from build123d import *

# Parameters (mm, degrees)
SKETCH1_W                   = 1212.85
SKETCH1_H                   = 736.6
BOSS_EXTRUDE1_DEPTH         = 6.35
H_0_266_DIAMETER_HOLE1_D    = 6.7564
H_0_266_DIAMETER_HOLE2_D    = 6.7564
H_0_266_DIAMETER_HOLE3_D    = 6.7564
SKETCH12_R                  = 3.175
CUT_EXTRUDE4_DEPTH          = 7.35
LPATTERN1_COUNT             = 5
LPATTERN1_PITCH             = 266.7
FILLET2_R                   = 3.175
CUT_EXTRUDE5_DEPTH          = 7.35
F_1_4_0_25_DIAMETER_HOLE1_D = 6.35


with BuildPart() as part:
    # Sketch1 → Boss-Extrude1 (new body)
    with BuildSketch(Plane.XY):
        Rectangle(SKETCH1_W, SKETCH1_H)
    extrude(amount=BOSS_EXTRUDE1_DEPTH)

    # H (0.266) Diameter Hole1 (through all)
    with Locations(Plane.XY.offset(6.35)):
        with Locations((-565.15, -342.9), (-158.75, -342.9), (247.65, -342.9)):
            Hole(H_0_266_DIAMETER_HOLE1_D / 2)

    # H (0.266) Diameter Hole2 (through all)
    with Locations(Plane.XY.offset(6.35)):
        with Locations((-582.6125, 323.596), (-582.6125, 171.196), (-582.6125, 18.796), (-582.6125, -133.604)):
            Hole(H_0_266_DIAMETER_HOLE2_D / 2)

    # H (0.266) Diameter Hole3 (through all)
    with Locations(Plane.XY.offset(6.35)):
        with Locations((223.770762516, 324.305909426), (436.157706379, 167.711380386), (301.059782944, 190.437399177)):
            Hole(H_0_266_DIAMETER_HOLE3_D / 2)

    # Sketch12 → Cut-Extrude4 (cut, through all)
    with BuildSketch(Plane.XY.offset(6.35)):
        with Locations((-536.575, 361.95)):
            Circle(SKETCH12_R)
        with BuildLine():
            Line((-552.45, 355.6), (-520.7, 355.6))
            ThreePointArc((-520.7, 355.6), (-508, 342.9), (-520.7, 330.2))
            Line((-520.7, 330.2), (-552.45, 330.2))
            ThreePointArc((-552.45, 330.2), (-565.15, 342.9), (-552.45, 355.6))
        make_face()
    cut_extrude4 = extrude(amount=-CUT_EXTRUDE4_DEPTH, mode=Mode.SUBTRACT)

    # LPattern1: Cut-Extrude4 ×5
    with Locations(*[(i * LPATTERN1_PITCH, 0, 0) for i in range(1, LPATTERN1_COUNT)]):
        add(cut_extrude4, mode=Mode.SUBTRACT)

    # Fillet2
    fillet2_edges = [part.edges().sort_by_distance(p)[0] for p in [
        (606.425, -368.3, 3.175),
        (-606.425, -368.3, 3.175),
        (-606.425, 368.3, 3.175),
        (606.425, 368.3, 3.175),
    ]]
    fillet(fillet2_edges, radius=FILLET2_R)

    # Sketch14 → Cut-Extrude5 (cut, through all)
    with BuildSketch(Plane.XY.offset(6.35)):
        with BuildLine():
            Line((336.240912114, 244.52397913), (412.150948109, 237.882711533))
            ThreePointArc((412.150948109, 237.882711533), (435.240537575, 210.365610336), (407.723436378, 187.27602087))
            Line((407.723436378, 187.27602087), (331.813400383, 193.917288467))
            ThreePointArc((331.813400383, 193.917288467), (308.723810917, 221.434389664), (336.240912114, 244.52397913))
        make_face()
    extrude(amount=-CUT_EXTRUDE5_DEPTH, mode=Mode.SUBTRACT)

    # 1/4 (0.25) Diameter Hole1 (through all)
    with Locations(Plane.XY.offset(6.35)):
        with Locations((596.9, -358.775), (596.9, -225.425), (596.9, -92.075)):
            Hole(F_1_4_0_25_DIAMETER_HOLE1_D / 2)


solid = part.part
CAD build for the part. Positions are in the model's coordinates, mm. Coordinates: 2 decimals unless noted, no trailing zeros. Loops run counter-clockwise (first coordinate to the right, second up) from the corner with the lowest first, then second, coordinate; pieces in that order, holes last. Notation, with made-up numbers: (21, 66) -> (70, 66) arc R13 cw to (70, 78) -> close; hole circle Ø4 at (81, 21.5). An arc over 180 degrees is marked (long way). One line per item, written item: value.
1. Slice it at A-A on y = 342.9. Write the cut outline in (x, z) (3 decimals).
Answers:
outline: (-606.425, 0) -> (-565.15, 0) -> (-565.15, 6.35) -> (-606.425, 6.35) -> close; (-508, 0) -> (-298.45, 0) -> (-298.45, 6.35) -> (-508, 6.35) -> close; (-241.3, 0) -> (-31.75, 0) -> (-31.75, 6.35) -> (-241.3, 6.35) -> close; (25.4, 0) -> (234.95, 0) -> (234.95, 6.35) -> (25.4, 6.35) -> close; (292.1, 0) -> (501.65, 0) -> (501.65, 6.35) -> (292.1, 6.35) -> close; (558.8, 0) -> (606.425, 0) -> (606.425, 6.35) -> (558.8, 6.35) -> close
2. Pull direction Y, two halves, no side cores. Call faces 1 (the face through (-8, 5, 0)), 2 (the face through (435.283, 210.923, 3.219)): pulls with the +Y half, pulls with the -Y half, needs draft (parallel to the pull), parting line crosses it, or undercut.
Answers:
face 1: needs draft
face 2: undercut
3. Drill centre lines: line 1 (X direction, y = 361.95, z = 2.75) (3 decimals); line 2 (Y direction, x = -543, z = 4.75); line 3 (X direction, y = 168.5, z = 5.25) (3 decimals). Where is each one in solid material? Low to high. Write a range as [from, to].
Answers:
line 1: x = [-606.425, -539.75], [-533.4, -273.05], [-266.7, -6.35], [0, 260.35], [266.7, 527.05], [533.4, 606.425]
line 2: y = [-368.3, 330.2], [355.6, 368.3]
line 3: x = [-606.425, -584.648], [-580.577, 432.873], [439.443, 606.425]
